The listing builds one solid part. Answer for the finished solid, in the listing's coordinates (mm). A direction names the side the tool comes from. Coordinates: 2 decimals unless noted, no trailing zeros. Order: outer loops, then holes, each group sorted by start corner. A loop starts at its lowest first (then second) coordinate and runs counter-clockwise, first axis right, second up.
from build123d import *

# Parameters (mm, degrees)
F0_W         = 62
F0_H         = 40
F0_R         = 2.25
F1_DEPTH     = 2
F2_W         = 46
F2_H         = 42
F2_R         = 1.7
F2_R_2       = 12
F3_DEPTH     = 2
F5_DEPTH     = 1.5
F6_R         = 2
F7_R         = 1
F8_T4_DEPTH  = 41.5
F8_T9_ANGLE  = 233.2969892374
F8_T15_ANGLE = 233.2969892374
F8_T21_DEPTH = 41.5


# Not quite as in the source:
# - a fillet or chamfer that OpenCascade refuses, or shapes differently, is made with other operations: its cross-section is extruded or revolved along the edge and cut away or added
# - a pattern or mirror of a feature is missing from the dataset's text; its kind, count and spacing are read off the source's solid


with BuildPart() as f1:
    # F0 (on Top) → F1 (new body)
    with BuildSketch(Plane.XY):
        with Locations((0, -20)):
            Rectangle(F0_W, F0_H)
        with Locations((-27, -35)):
            Circle(F0_R, mode=Mode.SUBTRACT)
        with Locations((27, -35)):
            Circle(F0_R, mode=Mode.SUBTRACT)
        with Locations((-27, -20)):
            Circle(F0_R, mode=Mode.SUBTRACT)
        with Locations((-27, -5)):
            Circle(F0_R, mode=Mode.SUBTRACT)
        with Locations((27, -20)):
            Circle(F0_R, mode=Mode.SUBTRACT)
        with Locations((27, -5)):
            Circle(F0_R, mode=Mode.SUBTRACT)
    extrude(amount=F1_DEPTH)

    # F2 (on Front) → F3 (join)
    with BuildSketch(Plane.XZ):
        with Locations((0, 23)):
            Rectangle(F2_W, F2_H)
        with Locations((-15.5, 7.5)):
            Circle(F2_R, mode=Mode.SUBTRACT)
        with Locations((15.5, 7.5)):
            Circle(F2_R, mode=Mode.SUBTRACT)
        with Locations((-15.5, 38.5)):
            Circle(F2_R, mode=Mode.SUBTRACT)
        with Locations((0, 23)):
            Circle(F2_R_2, mode=Mode.SUBTRACT)
        with Locations((15.5, 38.5)):
            Circle(F2_R, mode=Mode.SUBTRACT)
    extrude(amount=F3_DEPTH)

    # F4 (on face) → F5 (join)
    with BuildSketch(Plane.YZ.offset(23)):
        Polygon((-2, 2), (-2, 44), (-40, 2), align=None)
    f5 = extrude(amount=-F5_DEPTH)

    # F5_copies: F5 across plane
    add(f5.mirror(Plane(origin=(0, 0, 0), x_dir=(0, 0, -1), z_dir=(-1, 0, 0))))

    # F6
    f6_edges = [f1.edges().sort_by_distance(p)[0] for p in [
        (31, -40, 1),
        (31, 0, 1),
        (-31, 0, 1),
        (-31, -40, 1),
    ]]
    fillet(f6_edges, radius=F6_R)

    # F7
    f7_edges = [f1.edges().sort_by_distance(p)[0] for p in [
        (-23, 0, 23),
        (23, 0, 23),
    ]]
    fillet(f7_edges, radius=F7_R)

    # F8: fillet of radius 1 on 4 edges, made by hand


with BuildPart() as f8_tool2:
    # F8_s3 → F8_t4 (new body)
    with BuildSketch(Plane.XZ.offset(1)):
        with BuildLine():
            ThreePointArc((24, 2), (23.2928932188, 2.2928932188), (23, 3))
            Line((23, 3), (23, 2))
            Line((23, 2), (24, 2))
        make_face()
    extrude(amount=F8_T4_DEPTH)

    split(bisect_by=Plane(origin=(0, -22.9900249377, 20.8004987531), x_dir=(1, 0, 0), z_dir=(0, 0.7415357791, -0.670913324)), keep=Keep.TOP)


with BuildPart() as f1_1:
    add(f1.part)

    # F8_t1: union F8_tool2
    add(f8_tool2.part)


with BuildPart() as f8_tool7:
    # F8_s8 → F8_t9 (revolve)
    with BuildSketch(Plane(origin=(14.6206404523, -10.8990847056, 0), x_dir=(0, 0, 1), z_dir=(0.8017442393, -0.5976672776, 0))):
        with BuildLine():
            ThreePointArc((3, -11.3469358686), (2.2928932188, -11.0540426498), (2, -10.3469358686))
            Line((2, -10.3469358686), (2, -11.3469358686))
            Line((2, -11.3469358686), (3, -11.3469358686))
        make_face()
    revolve(axis=Axis((22, -1, 2), (0, 0, -1)), revolution_arc=F8_T9_ANGLE)

    split(bisect_by=Plane.XZ, keep=Keep.TOP)

    split(bisect_by=Plane.XZ.offset(2), keep=Keep.BOTTOM)


with BuildPart() as f1_2:
    add(f1_1.part)

    # F8_t6: union F8_tool7
    add(f8_tool7.part)


with BuildPart() as f8_tool13:
    # F8_s14 → F8_t15 (revolve)
    with BuildSketch(Plane(origin=(-14.6206404523, -10.8990847056, 0), x_dir=(0, 0, 1), z_dir=(-0.8017442393, -0.5976672776, 0))):
        with BuildLine():
            ThreePointArc((3, 11.3469358686), (2.2928932188, 11.0540426498), (2, 10.3469358686))
            Line((2, 10.3469358686), (2, 11.3469358686))
            Line((2, 11.3469358686), (3, 11.3469358686))
        make_face()
    revolve(axis=Axis((-22, -1, 2), (0, 0, 1)), revolution_arc=F8_T15_ANGLE)

    split(bisect_by=Plane.XZ, keep=Keep.TOP)

    split(bisect_by=Plane.XZ.offset(2), keep=Keep.BOTTOM)


with BuildPart() as f1_3:
    add(f1_2.part)

    # F8_t12: union F8_tool13
    add(f8_tool13.part)


with BuildPart() as f8_tool19:
    # F8_s20 → F8_t21 (new body)
    with BuildSketch(Plane.XZ.offset(1)):
        with BuildLine():
            ThreePointArc((-24, 2), (-23.2928932188, 2.2928932188), (-23, 3))
            Line((-23, 3), (-23, 2))
            Line((-23, 2), (-24, 2))
        make_face()
    extrude(amount=F8_T21_DEPTH)

    split(bisect_by=Plane(origin=(0, -22.9900249377, 20.8004987531), x_dir=(1, 0, 0), z_dir=(0, 0.7415357791, -0.670913324)), keep=Keep.TOP)


with BuildPart() as f1_4:
    add(f1_3.part)

    # F8_t18: union F8_tool19
    add(f8_tool19.part)


solid = f1_4.part
1) Section A-A (x = 27) is taken. Give the vertices of the cut face in (y, z).
2) A tool of negligible diameter and unlimited length cuts with its end or side. For faces 1 (the face through (-30, -20, 2)), 2 (the face through (30, -20, 2)), 3 (the face through (-21.5, -13, 14)), from which of +Z, -Z, +X, -X, +Y, -Y can it reach the whole face along a straight path? Write none if from no direction.
3) Section B-B (x = 15.5) is taken. Give the vertices of the cut face in (y, z), then the cut area to 3 significant figures.
4) Each of these flat-tipped pins is pushed along its axis until it touches: P1, Ø5, axis at x = -27, y = -35, coming from the +Z side; P2, Ø6, axis at y = -14.5, z = 9.5, coming from the -X side; P3, Ø2, axis at x = -17, z = 33, coming from the -Y side; P4, Ø3, axis at x = 15.5, z = 38.5, coming from the -Y side (3 decimals). Where does it stop, or does it pass through?
5) Consider L1, parallel to Y at x = 27, z = 1.6; L2, parallel to Z at x = -15.5, y = -0.8; L3, parallel to X at y = -24.5, z = 12.5. Determine where each line is inside the solid, lowest interval first.
6) Section C-C (z = 16) is taken. Give the vertices of the cut face in (x, y).
7) Determine the mould class of faces 4 (the face through (30.4, -0.57, 1.01)), 5 (the face through (28.038, -21.996, 0.986)), 6 (the face through (-24.854, -4.324, 0.986)), 7 (the face through (9, -2, 14)) for opening direction Y: released by +Y, released by -Y, zero draft, split by the parting line, or undercut.
8) Section D-D (y = -20) is taken. Give the vertices of the cut face in (x, z).
Filled sheet:
1. outline: (-40, 0) - (-37.25, 0) - (-37.25, 2) - (-40, 2) - close; (-32.75, 0) - (-22.25, 0) - (-22.25, 2) - (-32.75, 2) - close; (-17.75, 0) - (-7.25, 0) - (-7.25, 2) - (-17.75, 2) - close; (-2.75, 0) - (0, 0) - (0, 2) - (-2.75, 2) - close
2. face 1: +Z, -X, +Y, -Y
2. face 2: +Z, +X, +Y, -Y
2. face 3: +Z, -Y
3. outline: (-40, 0) - (0, 0) - (0, 5.8) - (-2, 5.8) - (-2, 2) - (-40, 2) - close; (-2, 9.2) - (0, 9.2) - (0, 36.8) - (-2, 36.8) - close; (-2, 40.2) - (0, 40.2) - (0, 44) - (-2, 44) - close
3. area: 150 mm2
4. P1: stops at z = 2
4. P2: stops at x = -23
4. P3: stops at y = -2
4. P4: passes through
5. L1: y = -40 to -37.25, -32.75 to -22.25, -17.75 to -7.25, -2.75 to 0
5. L2: z = 0 to 5.8, 9.2 to 36.8, 40.2 to 44
5. L3: x = -23 to -21.5, 21.5 to 23
6. outline: (-23, -27.33) - (-21.5, -27.33) - (-21.5, -2) - (-9.75, -2) - (-9.75, 0) - (-22, 0) arc R1 ccw to (-23, -1) - close; (9.75, -2) - (21.5, -2) - (21.5, -27.33) - (23, -27.33) - (23, -1) arc R1 ccw to (22, 0) - (9.75, 0) - close
7. face 4: released by +Y
7. face 5: undercut
7. face 6: undercut
7. face 7: released by -Y
8. outline: (-31, 0) - (-29.25, 0) - (-29.25, 2) - (-31, 2) - close; (-24.75, 0) - (24.75, 0) - (24.75, 2) - (24, 2) arc R1 cw to (23, 3) - (23, 24.11) - (21.5, 24.11) - (21.5, 2) - (-21.5, 2) - (-21.5, 24.11) - (-23, 24.11) - (-23, 3) arc R1 cw to (-24, 2) - (-24.75, 2) - close; (29.25, 0) - (31, 0) - (31, 2) - (29.25, 2) - close
